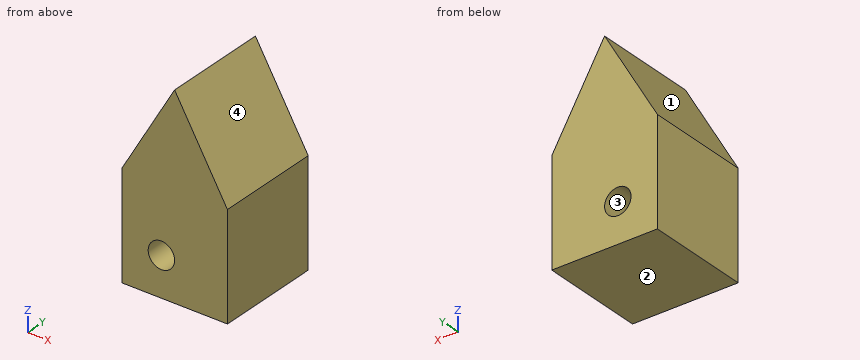
from build123d import *

# Parameters (mm, degrees)
F0_W     = 50.8
F0_H     = 50.8
F0_R     = 6.35
F1_DEPTH = 50.8


with BuildPart() as f1:
    # F0 (on Front) → F1 (new body)
    with BuildSketch(Plane.XZ):
        Polygon((0, 74.828401), (-25.4, 30.834311), (25.4, 30.834311), align=None)
        with Locations((0, 5.434311)):
            Rectangle(F0_W, F0_H)
        with Locations((-6.35, -0.915689)):
            Circle(F0_R, mode=Mode.SUBTRACT)
    extrude(amount=F1_DEPTH)


solid = f1.part
Model file for the job. Use its own axes, mm. Face numbers are marked on the shaded views. Give positions to 0.01 mm unless a question says otherwise; leave off trailing zeros. Loops run counter-clockwise (first coordinate to the right, second up) from the corner with the lowest first, then second, coordinate; pieces in that order, holes last. Notation, with made-up numbers: (34, 3.25) -> (58, 3.25) arc R23 cw to (58, 11.25) -> close; hole circle Ø6 at (26.25, -22.75). An arc over 180 degrees is marked (long way). Use a Markdown table: item, result. Add a question column.
(1) Mould opens along X. For the marked faces 1, 2, 3 and 4 say: +X half, -X half, draft (parallel to the pull), parting line (faces both ways), or undercut.
(2) Slice it at D-D on x = 14. List the corners of the cut face in (y, z).
(3) Drop a flat-ended pin along its axis: pin 1 Ø4 at (x, y) = (-4, -25.5) entering from +Z. Give the stop position or say it passes through.
(4) Slice it at C-C on z = 63. List the corners of the cut face in (x, y).
(5) Slice it at A-A on x = -6.35. List the corners of the cut face in (y, z), and give its area (3 significant figures).
(6) Slice it at B-B on y = -31. List the corners of the cut face in (x, z).
(7) Wall check: line 1 along Z through (x, y) = (-6, -10); line 2 along X through (y, z) = (-10, -4); line 3 along Z through (x, y) = (-6.35, -30). Give the ranges that are in metal, low to high.
Filled sheet:
| question | item | result |
|---|---|---|
| 1 | face 1 | -X half |
| 1 | face 2 | draft |
| 1 | face 3 | undercut |
| 1 | face 4 | +X half |
| 2 | outline | (-50.8, -19.97) -> (0, -19.97) -> (0, 50.58) -> (-50.8, 50.58) -> close |
| 3 | pin 1 | z = 71.36 |
| 4 | outline | (-6.83, -50.8) -> (6.83, -50.8) -> (6.83, 0) -> (-6.83, 0) -> close |
| 5 | outline | (-50.8, -19.97) -> (0, -19.97) -> (0, -7.27) -> (-50.8, -7.27) -> close; (-50.8, 5.43) -> (0, 5.43) -> (0, 63.83) -> (-50.8, 63.83) -> close |
| 5 | area | 3,610 mm2 |
| 6 | outline | (-25.4, -19.97) -> (25.4, -19.97) -> (25.4, 30.83) -> (0, 74.83) -> (-25.4, 30.83) -> close; hole circle Ø12.7 at (-6.35, -0.92) |
| 7 | line 1 | -19.97 to -7.26, 5.42 to 64.44 |
| 7 | line 2 | -25.4 to -11.9, -0.8 to 25.4 |
| 7 | line 3 | -19.97 to -7.27, 5.43 to 63.83 |
